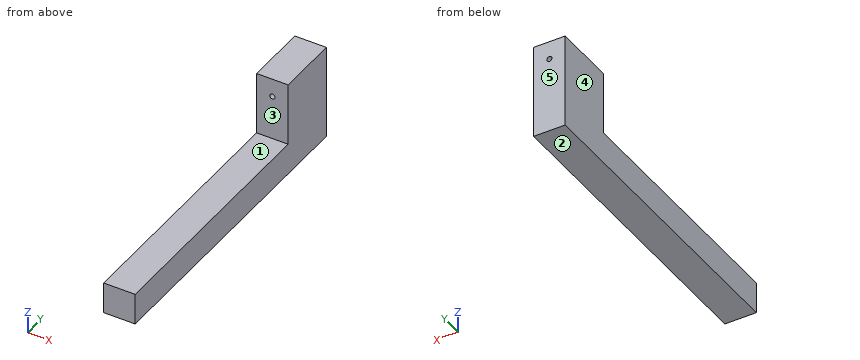
from build123d import *

# Parameters (mm, degrees)
SKETCH_W     = 15
SKETCH_H     = 15
PAD_DEPTH    = 150
SKETCH001_W  = 15
SKETCH001_H  = 30
PAD001_DEPTH = 30
SKETCH002_R  = 1.25
POCKET_DEPTH = 150.001


with BuildPart() as part:
    # Sketch → Pad (new body)
    with BuildSketch(Plane.XZ):
        Rectangle(SKETCH_W, SKETCH_H)
    extrude(amount=PAD_DEPTH)

    # Sketch001 (on Face3 of Pad) → Pad001 (join)
    with BuildSketch(Plane(origin=(0, 0, 7.5), x_dir=(-1, 0, 0), z_dir=(0, 0, 1))):
        with Locations((0, 15)):
            Rectangle(SKETCH001_W, SKETCH001_H)
    extrude(amount=PAD001_DEPTH)

    # Sketch002 → Pocket (cut, through all)
    with BuildSketch(Plane(origin=(0, 0, 0), x_dir=(1, 0, 0), z_dir=(0, 1, 0))):
        with Locations((0, -28.75)):
            Circle(SKETCH002_R)
    extrude(amount=-POCKET_DEPTH, mode=Mode.SUBTRACT)


solid = part.part
Check sheet for the modelled part. Datum: model origin and axes. Units: mm. Face numbers are marked on the shaded views. A direction names the side the tool comes from. Round coordinates to 2 decimals unless told otherwise and drop trailing zeros. Loops run counter-clockwise (first coordinate to the right, second up) from the corner with the lowest first, then second, coordinate; pieces in that order, holes last. Notation, with made-up numbers: M -22.75,-26.75 L -0.75,-26.75 A23 cw -0.75,12.25 Z; hole C -20,48.5 d3. An arc over 180 degrees is marked long. One line per question, with ' | ' between items. Start each with the question number.
Item 1: Gauge pin test, flat ends, axial feed: pin 1 Ø5 at (x, y) = (-5, -71) entering from +Z; pin 2 Ø4 at (x, z) = (0, 28.75) entering from +Y; pin 3 Ø2 at (x, z) = (-3.5, 25) entering from -Y. Record the tip position at first contact, or that the pin passes through.
Item 2: Scan lines: probe 1 along Z at (x, y) = (0, -15.25); probe 2 along X at (y, z) = (-8.5, 28.75); probe 3 along Z at (x, y) = (-1.75, -69). Record each from-to range of solid material in increasing order.
Item 3: Section check B-B (x = 4). Record the boundary of the cut face in (y, z).
Item 4: Set-up check for the marked faces 1 and 2: record each of +Z, -Z, +X, -X, +Y, -Y from which the full face is reachable in a straight line by a thin tool's end or side.
Item 5: Release check for a two-part mould opening along Y. For the marked faces 3, 4 and 5 record: released by +Y, released by -Y, zero draft, split by the parting line, or undercut.
Item 6: Section check C-C (z = 32.5). Record the boundary of the cut face in (x, y), and give its area (3 significant figures).
Item 7: Section check A-A (y = -117). Record the boundary of the cut face in (x, z).
Worked out:
1) pin 1: z = 7.5 | pin 2: y = 0 | pin 3: y = -30
2) probe 1: -7.5 to 27.5, 30 to 37.5 | probe 2: -7.5 to -1.25, 1.25 to 7.5 | probe 3: -7.5 to 7.5
3) outline: M -150,-7.5 L 0,-7.5 L 0,37.5 L -30,37.5 L -30,7.5 L -150,7.5 Z
4) face 1: +Z, +X, -X, -Y | face 2: -Z, +X, -X, +Y, -Y
5) face 3: released by -Y | face 4: zero draft | face 5: released by +Y
6) outline: M -7.5,-30 L 7.5,-30 L 7.5,0 L -7.5,0 Z | area: 450 mm^2
7) outline: M -7.5,-7.5 L 7.5,-7.5 L 7.5,7.5 L -7.5,7.5 Z
